Geometry check sheet. Reference: drawing and pictorial views, mm from the part's lowest x, y, z. A direction names the side the tool comes from. Give positions to 0.01 mm unless a question says otherwise; leave off trailing zeros. Loops run counter-clockwise (first coordinate to the right, second up) from the corner with the lowest first, then second, coordinate; pieces in that order, holes last. Notation, with made-up numbers: (57.25, 17.5) - (67.25, 17.5) arc R19 cw to (67.25, 24.5) - close; hole circle Ø2 at (64.5, -3.75). An arc over 180 degrees is marked (long way). One line per question, with ' | ' between items. Start each with the question number.
1. Mould release check, pull along X, two halves, no side actions. Record for the marked faces 4, 5 and 6: +X half, -X half, draft (parallel to the pull), parting line (faces both ways), or undercut.
2. Section check B-B, the plane y = 121.8. Enter the section's corners in (x, z).
3. Section check C-C, the plane x = 23. Enter the section's corners in (y, z) (1 decimal), then the cut area to 3 significant figures.
4. Depth check by flat-ended pin: pin 1 Ø6 at (y, z) = (50.5, 10) entering from +X; pin 2 Ø4.5 at (y, z) = (121.8, 10) entering from +X; pin 3 Ø2 at (x, z) = (22, 4) entering from -Y. Enter the tip coordinate at first touch or a pass-through.
5. Section check D-D, the plane z = 3. Enter the section's corners in (x, y).
6. Thickness scan on line 1 along Y through (x, z) = (41, 13.5); line 2 along Y through (x, z) = (45.5, 14.75); line 3 along X through (y, z) = (113.5, 7.75). Record the ranges inside material, lowest first. Write a range as from..to.
7. Tool access check on the marked faces 1, 2 and 3. Record the directions out of +Z, -Z, +X, -X, +Y, -Y that give a thin tool (end or side, any length) a straight path to the whole face; none if there is none.
8. Section check A-A, the plane z = 10. Enter the section's corners in (x, y), then the cut area to 3 significant figures.
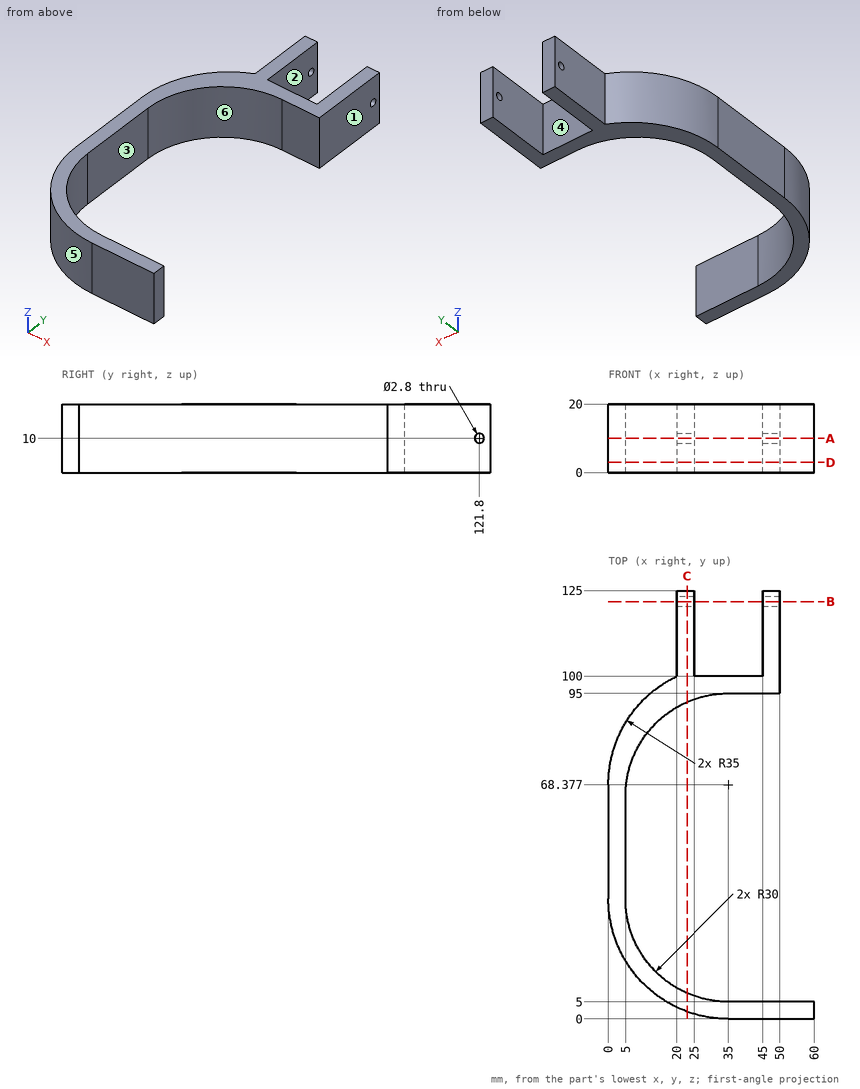
Results list:
1) face 4: undercut | face 5: -X half | face 6: +X half
2) outline: (20, 0) - (25, 0) - (25, 8.6) - (20, 8.6) - close; (20, 11.4) - (25, 11.4) - (25, 20) - (20, 20) - close; (45, 0) - (50, 0) - (50, 8.6) - (45, 8.6) - close; (45, 11.4) - (50, 11.4) - (50, 20) - (45, 20) - close
3) outline: (2.1, 0) - (7.5, 0) - (7.5, 20) - (2.1, 20) - close; (92.5, 0) - (125, 0) - (125, 20) - (92.5, 20) - close; hole circle Ø2.8 at (121.8, 10) | area: 752 mm²
4) pin 1: x = 5 | pin 2: x = 50 | pin 3: y = 2.12
5) outline: (0, 35) arc R35 ccw to (35, 0) - (60, 0) - (60, 5) - (35, 5) arc R30 cw to (5, 35) - (5, 65) arc R30 cw to (35, 95) - (50, 95) - (50, 125) - (45, 125) - (45, 100) - (25, 100) - (25, 125) - (20, 125) - (20, 100) arc R35 ccw to (0, 68.38) - close
6) line 1: 0..5, 95..100 | line 2: 0..5, 95..125 | line 3: 20..25, 45..50
7) face 1: +Z, -Z, +X, +Y | face 2: +Z, -Z, +Y | face 3: +Z, -Z, +X
8) outline: (0, 35) arc R35 ccw to (35, 0) - (60, 0) - (60, 5) - (35, 5) arc R30 cw to (5, 35) - (5, 65) arc R30 cw to (35, 95) - (50, 95) - (50, 120.4) - (45, 120.4) - (45, 100) - (25, 100) - (25, 120.4) - (20, 120.4) - (20, 100) arc R35 ccw to (0, 68.38) - close; (20, 123.2) - (25, 123.2) - (25, 125) - (20, 125) - close; (45, 123.2) - (50, 123.2) - (50, 125) - (45, 125) - close | area: 1,170 mm²
